from build123d import *

# Parameters (mm, degrees)
SKETCH_21_W         = 20
SKETCH_21_H         = 10
EXTRUDE_3_DEPTH     = 3
SKETCH_22_W         = 20
SKETCH_22_H         = 3
EXTRUDE_4_DEPTH     = 7
SKETCH_23_W         = 20
SKETCH_23_H         = 3
EXTRUDE_5_DEPTH     = 10
SKETCH_24_W         = 20
SKETCH_24_H         = 3
EXTRUDE_6_DEPTH     = 10
SKETCH_25_R         = 1.75
CUT_EXTRUDE_1_DEPTH = 21.976176963
SKETCH_26_R         = 3
SKETCH_26_R_2       = 1.75
CUT_EXTRUDE_2_DEPTH = 1
FILLET_1_R          = 1


with BuildPart() as part:
    # 草图21 → 凸台-拉伸3 (new body)
    with BuildSketch(Plane(origin=(0, 0, 0), x_dir=(1, 0, 0), z_dir=(0, 1, 0))):
        Rectangle(SKETCH_21_W, SKETCH_21_H)
    extrude(amount=EXTRUDE_3_DEPTH)

    # 草图22 → 凸台-拉伸4 (add)
    with BuildSketch(Plane(origin=(0, 3, 0), x_dir=(1, 0, 0), z_dir=(0, 1, 0))):
        with Locations((0, -6.5)):
            Rectangle(SKETCH_22_W, SKETCH_22_H)
        with Locations((0, 6.5)):
            Rectangle(SKETCH_22_W, SKETCH_22_H)
    extrude(amount=-EXTRUDE_4_DEPTH)

    # 草图23 → 凸台-拉伸5 (add)
    with BuildSketch(Plane.XY.offset(8)):
        with Locations((0, -2.5)):
            Rectangle(SKETCH_23_W, SKETCH_23_H)
    extrude(amount=EXTRUDE_5_DEPTH)

    # 草图24 → 凸台-拉伸6 (add)
    with BuildSketch(Plane(origin=(0, 0, -8), x_dir=(-1, 0, 0), z_dir=(0, 0, -1))):
        with Locations((0, -2.5)):
            Rectangle(SKETCH_24_W, SKETCH_24_H)
    extrude(amount=EXTRUDE_6_DEPTH)

    # 草图25 → 切除-拉伸1 (cut, through all)
    with BuildSketch(Plane(origin=(0, -1, 0), x_dir=(1, 0, 0), z_dir=(0, 1, 0))):
        with Locations(Location((-6, 14.5, 0), (0, 0, 270))):
            Circle(SKETCH_25_R)
        with Locations(Location((6, 14.5, 0), (0, 0, 270))):
            Circle(SKETCH_25_R)
        with Locations(Location((-6, -14.5, 0), (0, 0, 270))):
            Circle(SKETCH_25_R)
        with Locations(Location((6, -14.5, 0), (0, 0, 270))):
            Circle(SKETCH_25_R)
    extrude(amount=-CUT_EXTRUDE_1_DEPTH, mode=Mode.SUBTRACT)

    # 草图26 → 切除-拉伸2 (cut)
    # profile 1 of 4: a face of its own
    with BuildSketch(Plane(origin=(0, -1, 0), x_dir=(1, 0, 0), z_dir=(0, 1, 0))):
        with Locations(Location((-6, 14.5, 0), (0, 0, 270))):
            Circle(SKETCH_26_R)
        with Locations(Location((-6, 14.5, 0), (0, 0, 270))):
            Circle(SKETCH_26_R_2, mode=Mode.SUBTRACT)
    # profile 2 of 4: a face of its own
    with BuildSketch(Plane(origin=(0, -1, 0), x_dir=(1, 0, 0), z_dir=(0, 1, 0))):
        with Locations(Location((6, 14.5, 0), (0, 0, 270))):
            Circle(SKETCH_26_R)
        with Locations(Location((6, 14.5, 0), (0, 0, 270))):
            Circle(SKETCH_26_R_2, mode=Mode.SUBTRACT)
    # profile 3 of 4: a face of its own
    with BuildSketch(Plane(origin=(0, -1, 0), x_dir=(1, 0, 0), z_dir=(0, 1, 0))):
        with Locations(Location((-6, -14.5, 0), (0, 0, 270))):
            Circle(SKETCH_26_R)
        with Locations(Location((-6, -14.5, 0), (0, 0, 270))):
            Circle(SKETCH_26_R_2, mode=Mode.SUBTRACT)
    # profile 4 of 4: a face of its own
    with BuildSketch(Plane(origin=(0, -1, 0), x_dir=(1, 0, 0), z_dir=(0, 1, 0))):
        with Locations(Location((6, -14.5, 0), (0, 0, 270))):
            Circle(SKETCH_26_R)
        with Locations(Location((6, -14.5, 0), (0, 0, 270))):
            Circle(SKETCH_26_R_2, mode=Mode.SUBTRACT)
    extrude(amount=-CUT_EXTRUDE_2_DEPTH, mode=Mode.SUBTRACT)

    # 圆角1
    fillet_1_edges = [part.edges().sort_by_distance(p)[0] for p in [
        (10, -2.5, 18),
        (-10, -2.5, 18),
        (-10, -2.5, -18),
        (10, -2.5, -18),
        (0, 3, 8),
        (0, 3, -8),
        (0, -4, 5),
        (0, -4, -5),
    ]]
    fillet(fillet_1_edges, radius=FILLET_1_R)


solid = part.part
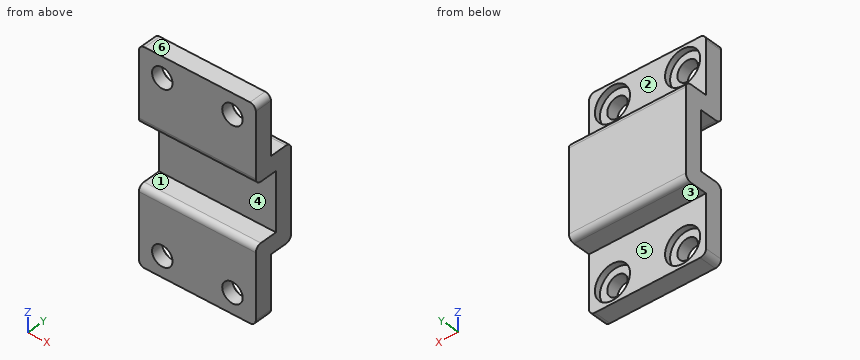
CAD build for the part. Positions are in the model's coordinates, mm. Face numbers are marked on the shaded views. A direction names the side the tool comes from. Give positions to 0.01 mm unless a question says otherwise; leave off trailing zeros. Write each loop counter-clockwise with the first axis right and the second up, starting at its lowest first coordinate (ties: lowest second). Pieces come first, ordered by that corner, then holes. Notation, with made-up numbers: (9, -23) -> (56, -23) arc R6 cw to (56, -16) -> close; hole circle Ø6 at (89, 4.25). An arc over 180 degrees is marked (long way). Return JSON: item names as keys, results as strings.
Item 1: Two-plate mould, pull along Z, no slides. Class the marked faces 4, 5 and 6: +Z half, -Z half, draft (parallel to the pull), parting line (faces both ways), or undercut.
Answer below:
{"face 4": "undercut", "face 5": "draft", "face 6": "+Z half"}
Item 2: Band-saw the part on A-A (z = 14.5). List the corners of the cut face in (x, y).
Answer below:
{"outline": "(-10, -4) -> (-7.75, -4) -> (-7.75, -2) -> (-9, -2) -> (-9, -1) -> (-10, -1) -> close; (-4.25, -4) -> (4.25, -4) -> (4.25, -2) -> (3, -2) -> (3, -1) -> (-3, -1) -> (-3, -2) -> (-4.25, -2) -> close; (7.75, -4) -> (10, -4) -> (10, -1) -> (9, -1) -> (9, -2) -> (7.75, -2) -> close"}
Item 3: Band-saw the part on D-D (y = 0.75). List the corners of the cut face in (x, z), then the cut area to 3 significant figures.
Answer below:
{"outline": "(-10, -8) -> (10, -8) -> (10, 8) -> (-10, 8) -> close", "area": "320 mm2"}
Item 4: Band-saw the part on C-C (x = -6). Give the number of separate pieces and of enclosed holes in the cut face, then the cut area to 3 significant figures.
Answer below:
{"separate pieces": "3", "enclosed holes": "0", "area": "105 mm2"}
Item 5: Drop flat-ended pins along their axis: pin 1 (8 mm diameter, centred on x = 2, z = -12.5, fed in from +Y); pin 2 (4 mm diameter, centred on x = 6, z = 14.5, fed in from +Y); pin 3 (3 mm diameter, centred on x = -1, z = -2.5, fed in from -Y). Give the stop position or say it passes through.
Answer below:
{"pin 1": "stops at y = -1", "pin 2": "stops at y = -2", "pin 3": "stops at y = 0"}
Item 6: Drill centre lines: probe 1 along X at (y, z) = (-1.55, 14.5); probe 2 along X at (y, z) = (-2.95, 14.5); probe 3 along Z at (x, y) = (5, -2.5). Where is each one in solid material? Low to high.
Answer below:
{"probe 1": "x = -10 to -9, -3 to 3, 9 to 10", "probe 2": "x = -10 to -7.75, -4.25 to 4.25, 7.75 to 10", "probe 3": "z = -18 to -15.94, -13.06 to -5, 5 to 13.06, 15.94 to 18"}
Item 7: Band-saw the part on B-B (x = 0.75). List the corners of the cut face in (y, z), then the cut area to 3 significant figures.
Answer below:
{"outline": "(-4, -18) -> (-1, -18) -> (-1, -8) -> (2, -8) arc R1 ccw to (3, -7) -> (3, 7) arc R1 ccw to (2, 8) -> (-1, 8) -> (-1, 18) -> (-4, 18) -> (-4, 6) arc R1 ccw to (-3, 5) -> (0, 5) -> (0, -5) -> (-3, -5) arc R1 ccw to (-4, -6) -> close", "area": "131 mm2"}
Item 8: Tool access for the marked faces 1, 2 and 3: list every direction of +Z, -Z, +X, -X, +Y, -Y with a clear straight run to the whole face (end or side of a thin tool).
Answer below:
{"face 1": "+X, -X, -Y", "face 2": "+Z, +X, -X, +Y", "face 3": "-Z, +X, -X, +Y"}
